Verification items for the finished model (mm, model axes). Give positions to 0.01 mm unless a question says otherwise; leave off trailing zeros. Loops run counter-clockwise (first coordinate to the right, second up) from the corner with the lowest first, then second, coordinate; pieces in that order, holes last. Notation, with made-up numbers: (87.25, 28.5) - (91.25, 28.5) arc R34 ccw to (91.25, 61.5) - close; hole circle Ø5 at (8, 36). An arc over 180 degrees is marked (long way). Use one line per item in the form item = value.
```python
from build123d import *

# Parameters (mm, degrees)
BASE_EXTRUDE_DEPTH = 1.5875
SKETCH2_R          = 3.3655
CUT_EXTRUDE1_DEPTH = 2.5875
LPATTERN1_COUNT    = 3
LPATTERN1_PITCH    = 0.79375


with BuildPart() as part:
    # Sketch1 → Base-Extrude (new body)
    with BuildSketch(Plane.XY):
        Polygon((5.499261314, 0), (2.749630657, 4.7625), (-2.749630657, 4.7625), (-5.499261314, 0), (-2.749630657, -4.7625), (2.749630657, -4.7625), align=None)
    extrude(amount=BASE_EXTRUDE_DEPTH)

    # Sketch2 → Cut-Extrude1 (cut, through all)
    with BuildSketch(Plane.XY.offset(1.5875)):
        Circle(SKETCH2_R)
    extrude(amount=-CUT_EXTRUDE1_DEPTH, mode=Mode.SUBTRACT)

    # Sketch3 → Cut-Revolve1 (revolve, cut)
    with BuildSketch(Plane(origin=(0, 0, 0), x_dir=(0, 0, 1), z_dir=(-0.866025404, 0.5, 0))):
        Polygon((1.3335, 5.499261314), (1.5875, 5.499261314), (1.5875, 4.799261314), align=None)
    cut_revolve1 = revolve(axis=Axis((0, 0, 0), (0, 0, 1)), mode=Mode.SUBTRACT)

    # Mirror1: Cut-Revolve1 across plane
    add(cut_revolve1.mirror(Plane.XY.offset(0.79375)), mode=Mode.SUBTRACT)

    # Sketch4 → Cut-Revolve2 (revolve, cut)
    with BuildSketch(Plane(origin=(0, 0, 0), x_dir=(0, 0, 1), z_dir=(-0.866025404, 0.5, 0))):
        Polygon((1.5875, 3.96875), (1.190625, 3.281342336), (1.984375, 3.281342336), align=None)
    cut_revolve2 = revolve(axis=Axis((0, 0, 0), (0, 0, 1)), mode=Mode.SUBTRACT)

    # LPattern1: Cut-Revolve2 ×3
    with Locations(*[(0, 0, -i * LPATTERN1_PITCH) for i in range(1, LPATTERN1_COUNT)]):
        add(cut_revolve2, mode=Mode.SUBTRACT)


solid = part.part
```
1. Scan lines: probe 1 along Y at (x, z) = (0, 0.4); probe 2 along Z at (x, y) = (3.5, -0.5); probe 3 along Z at (x, y) = (-2.5, 2.75). Record each from-to range of solid material in increasing order.
Result set:
probe_1 = -4.76 to -3.37, 3.37 to 4.76
probe_2 = 0.25 to 0.54, 1.04 to 1.34
probe_3 = 0.15 to 0.65, 0.94 to 1.44
2. Section check A-A, the plane x = 0. Record the cut outline in (y, z).
Result set:
outline = (-4.76, 0) - (-3.97, 0) - (-3.37, 0.35) - (-3.37, 0.45) - (-3.97, 0.79) - (-3.37, 1.14) - (-3.37, 1.24) - (-3.97, 1.59) - (-4.76, 1.59) - close; (3.37, 0.35) - (3.97, 0) - (4.76, 0) - (4.76, 1.59) - (3.97, 1.59) - (3.37, 1.24) - (3.37, 1.14) - (3.97, 0.79) - (3.37, 0.45) - close
3. Section check B-B, the plane x = -4.25. Record the cut outline in (y, z), then the cut area to 3 significant figures.
Result set:
outline = (-2.16, 0) - (2.16, 0) - (2.16, 1.59) - (-2.16, 1.59) - close
area = 6.87 mm²
4. Depth check by flat-ended pin: pin 1 Ø2 at (x, y) = (-1.5, 3.5) entering from -Z. Enter the tip coordinate at first touch or a pass-through.
Result set:
pin_1 = 0
